Here's the drawing with two shaded views (mm, measured from the low corner). I have some questions. A direction names the side the tool comes from. Round coordinates to 2 decimals unless told otherwise and drop trailing zeros. Order: outer loops, then holes, each group sorted by start corner. A loop starts at its lowest first (then second) coordinate and runs counter-clockwise, first axis right, second up. Notation, with made-up numbers: (49.5, 60) -> (86.5, 60) arc R27 cw to (86.5, 85) -> close; hole circle Ø1 at (45, -24). An arc over 180 degrees is marked (long way). One line per question, with ' | ' between items.
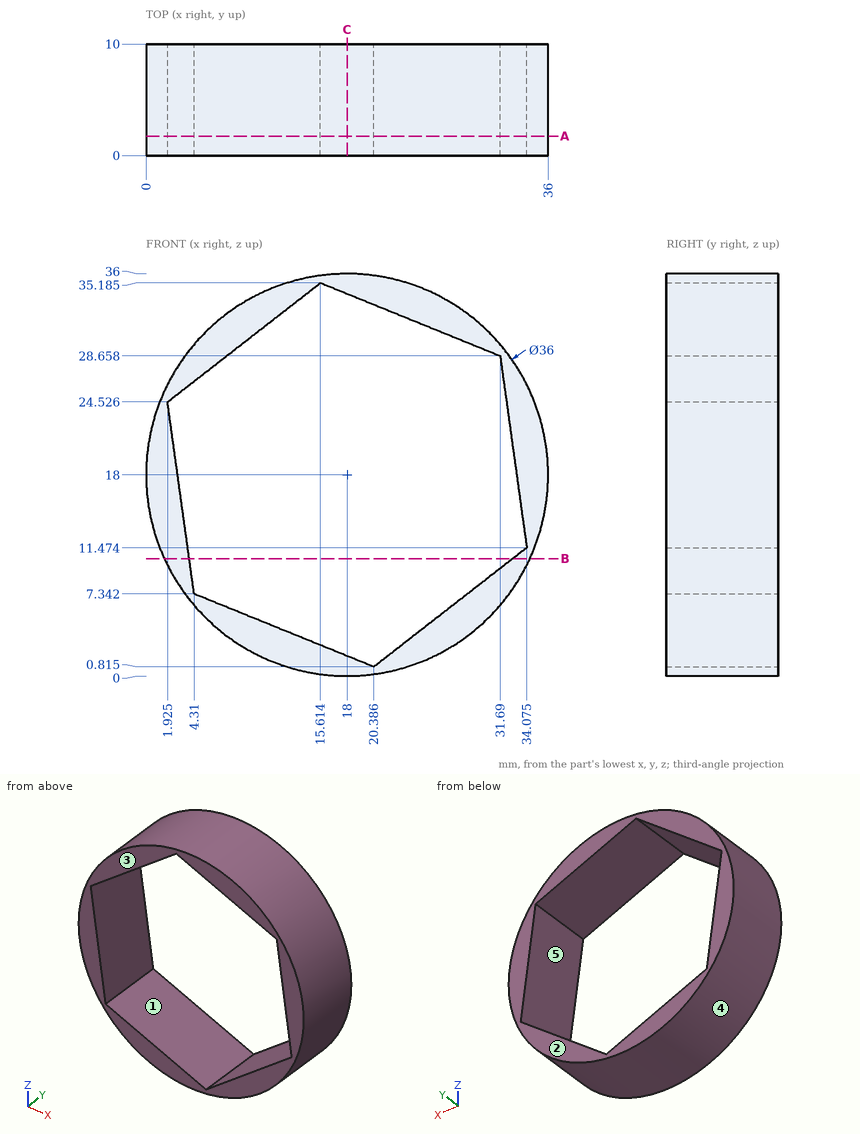
1. I need wall thicknesses on probe 1 along Z at (x, y) = (29, 7); probe 2 along Z at (x, y) = (10, 5.5) (1 decimal); probe 3 along X at (y, z) = (1.25, 32) (1 decimal). Which ranges of each line are inside material? Lowest first, please.
From the geometry:
probe 1: z = 3.75 to 7.52, 29.75 to 32.25 | probe 2: z = 1.9 to 5, 30.8 to 34.1 | probe 3: x = 6.7 to 11.5, 23.5 to 29.3
2. I'm going to push flat-ended pins straight in: pin 1 (10 mm diameter, centred on x = 8.5, z = 31, fed in from -Y); pin 2 (6 mm diameter, centred on y = 1.5, z = 28.5, fed in from +X); pin 3 (1.5 mm diameter, centred on x = 24, y = 1.5, fed in from +Z); pin 4 (1.5 mm diameter, centred on y = 8.5, z = 7, fed in from -X) (1 decimal). Where does each tip first touch, or does it pass through?
From the geometry:
pin 1: stops at y = 0 | pin 2: stops at x = 34.36 | pin 3: stops at z = 35.22 | pin 4: stops at x = 3.2
3. On a 3-axis mill with a long thin cutter (end or side, diameter ignored), from which of +Z, -Z, +X, -X, +Y, -Y can I reach the whole of each face in a straight line? I mean the marked faces 1 and 2. Say none if no direction works.
From the geometry:
face 1: +Y, -Y | face 2: +Z, -Z, +X, -X, +Y
4. I want a section at A-A on y = 1.75. List the corners of the cut face in (x, z) for me (1 decimal), and give its area (3 significant figures).
From the geometry:
outline: circle Ø36 at (18, 18); hole (1.9, 24.5) -> (4.3, 7.3) -> (20.4, 0.8) -> (34.1, 11.5) -> (31.7, 28.7) -> (15.6, 35.2) -> close | area: 236 mm²
5. I want a section at C-C on x = 18. List the corners of the cut face in (y, z) for me.
From the geometry:
outline: (0, 0) -> (10, 0) -> (10, 1.78) -> (0, 1.78) -> close; (0, 34.22) -> (10, 34.22) -> (10, 36) -> (0, 36) -> close
6. I want a section at B-B on z = 10.5. List the corners of the cut face in (x, y) for me (1 decimal).
From the geometry:
outline: (1.6, 0) -> (3.9, 0) -> (3.9, 10) -> (1.6, 10) -> close; (32.8, 0) -> (34.4, 0) -> (34.4, 10) -> (32.8, 10) -> close
7. If we mould it in two halves opening along X, with no side actions, what happens to the marked faces 3, 4 and 5? For each: pulls with the +X half, pulls with the -X half, needs draft (parallel to the pull), parting line crosses it, or undercut.
From the geometry:
face 3: needs draft | face 4: parting line crosses it | face 5: undercut
